```python
from build123d import *

# Parameters (mm, degrees)
F0_R          = 8
F0_R_2        = 6
F1_DEPTH      = 3
F0_R_3        = 10
F2_DEPTH      = 4
F3_DEPTH      = 25
F4_START      = 18
F4_DEPTH      = 4
F5_R          = 0.99999
F6_R          = 4.5
F7_DEPTH      = 25
F7_DEPTH_BACK = 25


# Not quite as in the source:
# - a fillet or chamfer is up to 0.001 mm smaller than in the source, because OpenCascade refuses the exact size


with BuildPart() as f1:
    # F0 (on Top) → F1 (new body)
    with BuildSketch(Plane.XY):
        Circle(F0_R)
        Circle(F0_R_2, mode=Mode.SUBTRACT)
    extrude(amount=-F1_DEPTH)

    # F0 (on Top) → F2 (join)
    with BuildSketch(Plane.XY):
        Circle(F0_R_3)
        Circle(F0_R, mode=Mode.SUBTRACT)
        Circle(F0_R)
        Circle(F0_R_2, mode=Mode.SUBTRACT)
    extrude(amount=F2_DEPTH)

    # F3 (add): a face of the model
    f3_faces = [f1.faces().sort_by_distance(p)[0] for p in [
        (-7.77372583, 0, -3),
    ]]
    extrude(f3_faces, amount=-F3_DEPTH)

    # F0 (on Top) → F4 (join)
    with BuildSketch(Plane.XY.offset(F4_START)):
        Circle(F0_R_2)
    extrude(amount=F4_DEPTH)

    # F5 (radius 1 in the source; OpenCascade refuses exactly that, so slightly less here)
    f5_edges = [f1.edges().sort_by_distance(p)[0] for p in [
        (-8, 0, 4),
        (-10, 0, 4),
        (-8, 0, 22),
    ]]
    fillet(f5_edges, radius=F5_R)

    # F6 (on face) → F7 (cut, two sides)
    with BuildSketch(Plane.XY.offset(22)) as f7_sk:
        Circle(F6_R)
    extrude(amount=-F7_DEPTH, mode=Mode.SUBTRACT)
    extrude(f7_sk.sketch, amount=F7_DEPTH_BACK, mode=Mode.SUBTRACT)


solid = f1.part
```
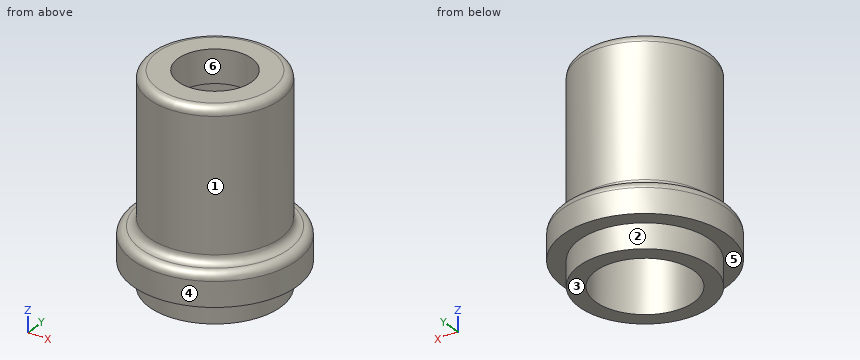
The listing builds one solid part. Answer for the finished solid, in the listing's coordinates (mm). Face numbers are marked on the shaded views. A direction names the side the tool comes from. Coordinates: 2 decimals unless noted, no trailing zeros. Write each loop counter-clockwise with the first axis right and the second up, starting at its lowest first coordinate (ties: lowest second). Pieces come first, ordered by that corner, then holes. Notation, with made-up numbers: (-28, -10.75) - (5, -10.75) arc R9 cw to (5, -2.75) - close; hole circle Ø4 at (40.25, 15). An arc over 180 degrees is marked (long way). Return JSON: item names as keys, results as strings. Group by question number.
Q1. Find the intervals of material crossed by line 1 along Y through (x, z) = (0, 9.25); line 2 along Y through (x, z) = (0, 20.3); line 3 along Z through (x, y) = (5, -5), in increasing order. Write a range as [from, to].
Q2. The part is cut by section D-D on z = 1.25. Write down the section's boundary in (x, y).
Q3. For a pull along Y with two mould halves and no side action, classify the marked faces 4, 5 and 6 as +Y half, -Y half, draft (parallel to the pull), parting line (faces both ways), or undercut.
Q4. Which of the six approach directions +Z, -Z, +X, -X, +Y, -Y give full straight-line access (tool end or side, diameter ignored) to the marked faces 1, 2 and 3?
Q5. Flat-ended cylindrical pins translate along their axes: pin 1 Ø9.5 at (x, y) = (2, 0) entering from -Z; pin 2 Ø6 at (x, z) = (-2.5, 15) entering from +Y; pin 3 Ø5 at (x, z) = (-0.5, 12) entering from -Y; pin 4 Ø3 at (x, y) = (0.5, 2) entering from +Z (3 decimals). Find the tip coordinate at first contact, or state that the pin passes through.
Q6. The part is cut by section C-C on z = 14.75. Write down the section's boundary in (x, y).
Evaluation:
{
 "1": {"line 1": "y = [-8, -6], [6, 8]", "line 2": "y = [-8, -4.5], [4.5, 8]", "line 3": "z = [-3, 22]"},
 "2": {"outline": "circle Ø20 at (0, 0); hole circle Ø12 at (0, 0)"},
 "3": {"face 4": "parting line", "face 5": "draft", "face 6": "undercut"},
 "4": {"face 1": "+Z", "face 2": "-Z", "face 3": "-Z, +X, -X, +Y, -Y"},
 "5": {"pin 1": "stops at z = -3", "pin 2": "stops at y = 8", "pin 3": "stops at y = -8", "pin 4": "passes through"},
 "6": {"outline": "circle Ø16 at (0, 0); hole circle Ø12 at (0, 0)"}
}
